from build123d import *

# Parameters (mm, degrees)
BOSS_EXTRUDE1_DEPTH = 4.826
SKETCH2_W           = 25.4
SKETCH2_H           = 4.826
CUT_EXTRUDE1_DEPTH  = 4.826


with BuildPart() as part:
    # Sketch1 → Boss-Extrude1 (new body)
    with BuildSketch(Plane.XY):
        Polygon((0, 76.2), (0, 101.6), (4.826, 101.6), (4.826, 127), (90.424, 127), (90.424, 101.6), (95.25, 101.6), (95.25, 76.2), (90.424, 76.2), (90.424, 50.8), (95.25, 50.8), (95.25, 25.4), (90.424, 25.4), (90.424, 0), (4.826, 0), (4.826, 25.4), (0, 25.4), (0, 50.8), (4.826, 50.8), (4.826, 76.2), align=None)
    extrude(amount=BOSS_EXTRUDE1_DEPTH)

    # Sketch2 → Cut-Extrude1 (cut)
    with BuildSketch(Plane(origin=(0, 127, 0), x_dir=(1, 0, 0), z_dir=(0, 1, 0))):
        with Locations((73.025, -2.413)):
            Rectangle(SKETCH2_W, SKETCH2_H)
        with Locations((22.225, -2.413)):
            Rectangle(SKETCH2_W, SKETCH2_H)
    extrude(amount=-CUT_EXTRUDE1_DEPTH, mode=Mode.SUBTRACT)


solid = part.part
Design review of the part built by this model. Coordinates are the model's own, in mm. A direction names the side the tool comes from. Give positions to 0.01 mm unless a question says otherwise; leave off trailing zeros. Loops run counter-clockwise (first coordinate to the right, second up) from the corner with the lowest first, then second, coordinate; pieces in that order, holes last. Notation, with made-up numbers: (63, 1) - (70, 1) arc R28 ccw to (70, 20) - close; hole circle Ø7 at (-15.5, -32.75). An arc over 180 degrees is marked (long way). Use CSV: the item, a comma, the result in double quotes. Start each with the question number.
1. Draft analysis for pull direction Y (two halves, no side actions). For faces 4 (the flat face through (93, 76.2, 2)), 5 (the flat face through (93, 101.6, 2)), 6 (the flat face through (0, 38, 2)), state which applies: released by +Y, released by -Y, zero draft, split by the parting line, or undercut.
2. Add section B-B (y = 115). State the section outline as (x, z) points, plus the area to 3 significant figures.
3. Insertion check: P1, Ø2.5, axis at y = 114.5, z = 3, coming from the +X side; P2, Ø2.5, axis at x = 93.5, z = 2, coming from the -Y side; P3, Ø2.5, axis at x = 93.5, z = 3, coming from the +Y side. Each pin has a flat end and moves straight along its axis. Give the tip position at first contact, or say it passes through.
4. Add section A-A (z = 2.9). State the section outline as (x, y) points (3 decimals).
5. Add section C-C (x = 23). State the section outline as (y, z) points.
6. Wall thickness on L1, parallel to Y at x = 69, z = 1.5; L2, parallel to X at y = 110, z = 1.55: over which ranges is each line inside the solid? List them lowest first.
7. Machinability: for faces 1 (the flat face through (73, 122.174, 2)), 2 (the flat face through (2, 50.8, 2)), 3 (the flat face through (90.424, 13, 2)), which of the approach directions +Z, -Z, +X, -X, +Y, -Y give a long, thin tool a straight path to every point of the face, cutting with its end or side? Answer none if there is none.
Results found:
1,face 4,"undercut"
1,face 5,"released by +Y"
1,face 6,"zero draft"
2,outline,"(4.83, 0) - (90.42, 0) - (90.42, 4.83) - (4.83, 4.83) - close"
2,area,"413 mm²"
3,P1,"stops at x = 90.42"
3,P2,"stops at y = 25.4"
3,P3,"stops at y = 101.6"
4,outline,"(0, 25.4) - (4.826, 25.4) - (4.826, 0) - (90.424, 0) - (90.424, 25.4) - (95.25, 25.4) - (95.25, 50.8) - (90.424, 50.8) - (90.424, 76.2) - (95.25, 76.2) - (95.25, 101.6) - (90.424, 101.6) - (90.424, 127) - (85.725, 127) - (85.725, 122.174) - (60.325, 122.174) - (60.325, 127) - (34.925, 127) - (34.925, 122.174) - (9.525, 122.174) - (9.525, 127) - (4.826, 127) - (4.826, 101.6) - (0, 101.6) - (0, 76.2) - (4.826, 76.2) - (4.826, 50.8) - (0, 50.8) - close"
5,outline,"(0, 0) - (122.17, 0) - (122.17, 4.83) - (0, 4.83) - close"
6,L1,"y = 0 to 122.17"
6,L2,"x = 4.83 to 90.42"
7,face 1,"+Z, -Z, +Y"
7,face 2,"+Z, -Z, -X"
7,face 3,"+Z, -Z, +X, -Y"
